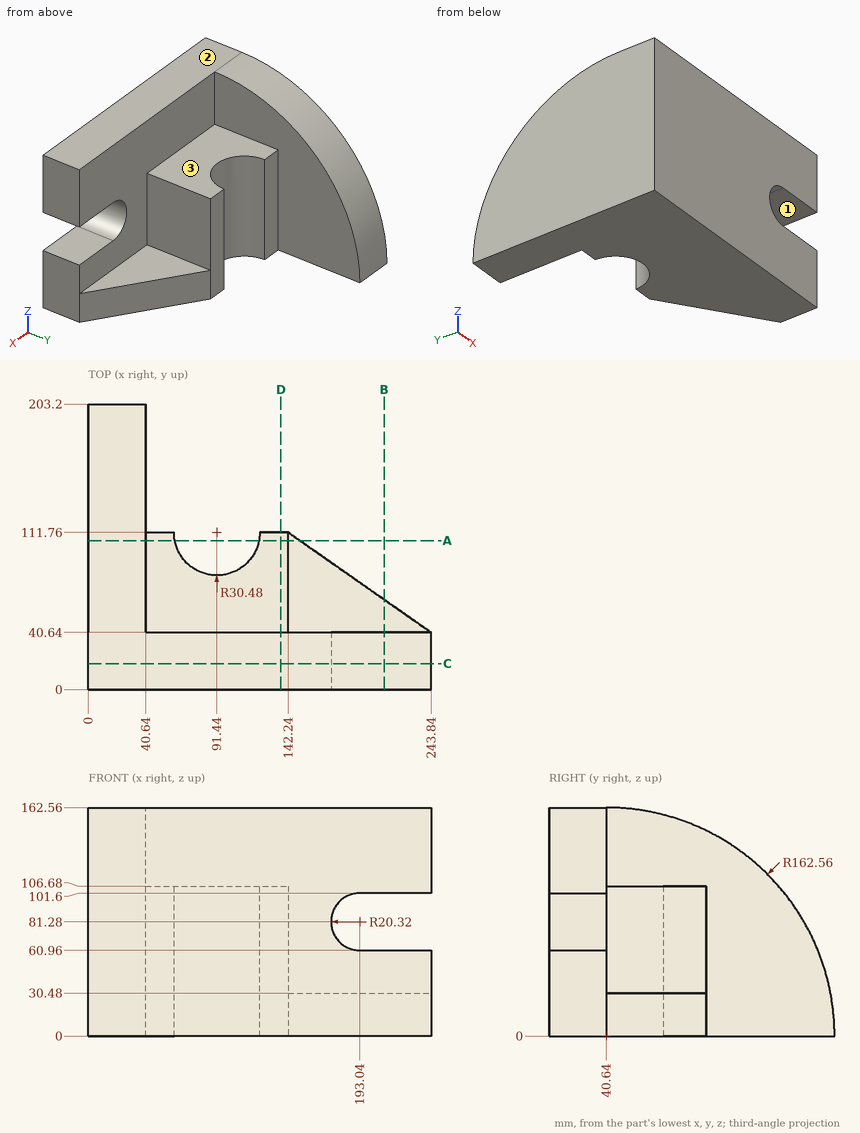
For this review, use the dimensioned drawing (mm, ordinates from the lowest corner) and the shaded views. A direction names the side the tool comes from. Give positions to 0.01 mm unless a question says otherwise; leave off trailing zeros. Loops run counter-clockwise (first coordinate to the right, second up) from the corner with the lowest first, then second, coordinate; pieces in that order, holes last. Notation, with made-up numbers: (43, 72) -> (91, 72) arc R24 ccw to (91, 98) -> close; hole circle Ø3 at (75.5, 38.25). An arc over 180 degrees is marked (long way). Use CSV: the item, a comma, the result in double quotes.
1. Machinability: for the marked faces 1, 2 and 3, which of the approach directions +Z, -Z, +X, -X, +Y, -Y give a long, thin tool a straight path to every point of the face, cutting with its end or side? Answer none if there is none.
Result:
face 1,"+X, +Y, -Y"
face 2,"+Z, +X, -X, +Y, -Y"
face 3,"+Z, +X, +Y"
2. Consider section D-D, the plane x = 137. Write out the cut boundary in (y, z), then the cut area to 3 significant figures.
Result:
outline,"(0, 0) -> (111.76, 0) -> (111.76, 106.68) -> (40.64, 106.68) -> (40.64, 162.56) -> (0, 162.56) -> close"
area,"14,200 mm²"
3. Consider section C-C, the plane y = 18.5. Write out the cut boundary in (x, z), then the cut area to 3 significant figures.
Result:
outline,"(0, 0) -> (243.84, 0) -> (243.84, 60.96) -> (193.04, 60.96) arc R20.32 cw to (193.04, 101.6) -> (243.84, 101.6) -> (243.84, 162.56) -> (0, 162.56) -> close"
area,"36,900 mm²"
4. Consider section B-B, the plane x = 210.5. Write out the cut boundary in (y, z).
Result:
outline,"(0, 0) -> (63.98, 0) -> (63.98, 30.48) -> (40.64, 30.48) -> (40.64, 60.96) -> (0, 60.96) -> close; (0, 101.6) -> (40.64, 101.6) -> (40.64, 162.56) -> (0, 162.56) -> close"
5. Consider section A-A, the plane y = 106. Write out the cut boundary in (x, z), then the cut area to 3 significant figures.
Result:
outline,"(0, 0) -> (61.51, 0) -> (61.51, 106.68) -> (40.64, 106.68) -> (40.64, 148.84) -> (0, 148.84) -> close; (121.37, 0) -> (150.47, 0) -> (150.47, 30.48) -> (142.24, 30.48) -> (142.24, 106.68) -> (121.37, 106.68) -> close"
area,"10,800 mm²"
6. To check wall thickness, follow probe 1 along X at (y, z) = (59, 100.5); probe 2 along X at (y, z) = (143, 96.5); probe 3 along Y at (x, z) = (92.5, 57.5). State the ranges of each line that lie inside material, in increasing order. Write a range as from..to.
Result:
probe 1,"x = 0..142.24"
probe 2,"x = 0..40.64"
probe 3,"y = 0..81.3"
7. For P1, Ø4, axis at y = 126.5, z = 88, coming from the +X side; P2, Ø10, axis at x = 47.5, z = 67, coming from the +Y side, all flat-tipped, find the tip position at first contact; note any pin that passes through.
Result:
P1,"stops at x = 40.64"
P2,"stops at y = 111.76"
